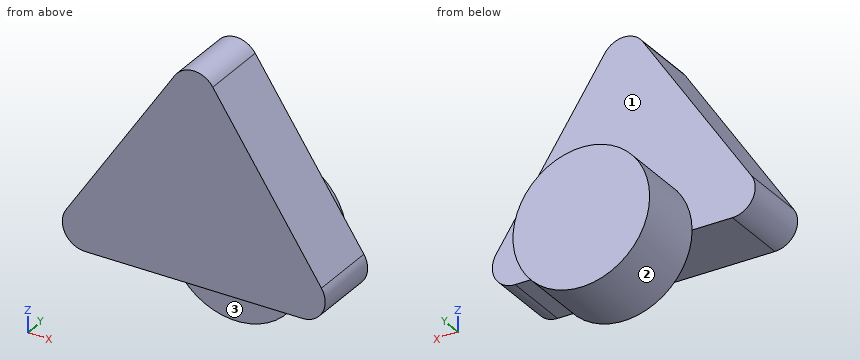
```python
from build123d import *

# Parameters (mm, degrees)
F1_DEPTH = 15
F2_R     = 15
F3_DEPTH = 15
F4_R     = 5
F5_R     = 5


with BuildPart() as f1:
    # F0 (on Front) → F1 (new body)
    with BuildSketch(Plane.XZ):
        Polygon((0, 50), (-33.166248, 0), (33.166248, 0), align=None)
    extrude(amount=F1_DEPTH)

    # F2 (on face) → F3 (join)
    with BuildSketch(Plane(origin=(0, 0, 0), x_dir=(-1, 0, 0), z_dir=(0, 1, 0))):
        Circle(F2_R)
    extrude(amount=F3_DEPTH)

    # F4
    f4_edges = [f1.edges().sort_by_distance(p)[0] for p in [
        (0, -7.5, 50),
    ]]
    fillet(f4_edges, radius=F4_R)

    # F5
    f5_edges = [f1.edges().sort_by_distance(p)[0] for p in [
        (33.166248, -7.5, 0),
        (-33.166248, -7.5, 0),
    ]]
    fillet(f5_edges, radius=F5_R)


solid = f1.part
```
CAD build for the part. Positions are in the model's coordinates, mm. Face numbers are marked on the shaded views. A direction names the side the tool comes from. Round coordinates to 2 decimals unless told otherwise and drop trailing zeros. Write each loop counter-clockwise with the first axis right and the second up, starting at its lowest first coordinate (ties: lowest second). Pieces come first, ordered by that corner, then holes. Notation, with made-up numbers: M -33.5,21.5 L 5.5,21.5 A32 cw 5.5,60.5 Z; hole C -30.5,70.25 d11. An arc over 180 degrees is marked long. One line per question, with ' | ' between items.
1. Cut at A-A on y = -12.5. Write the cut outline in (x, z).
Working result:
outline: M -28.02,7.76 A5 ccw -23.85,0 L 23.85,0 A5 ccw 28.02,7.76 L 4.17,43.72 A5 ccw -4.17,43.72 Z
2. Which spindle directions (+Z, -Z, +X, -X, +Y, -Y) get a long thin tool onto all of the face, cutting with end or side? Do the marked faces 1, 2 and 3. Say none if no direction does.
Working result:
face 1: +Z, +Y | face 2: +Y | face 3: -Z, +X, -X, -Y
3. Cut at D-D on x = -22.5. Write the cut outline in (y, z), and give its area (3 significant figures).
Working result:
outline: M -15,0 L 0,0 L 0,16.08 L -15,16.08 Z | area: 241 mm2
4. Pin check, flat tips, straight feed: pin 1 Ø4.5 at (x, y) = (7, -11) entering from -Z; pin 2 Ø10 at (y, z) = (-5.5, 27) entering from +X; pin 3 Ø10 at (y, z) = (-3.5, 3) entering from +X; pin 4 Ø3 at (x, z) = (0.5, 24.5) entering from +Y. Stop position of each tip, or through.
Working result:
pin 1: z = 0 | pin 2: x = 18.57 | pin 3: x = 28.85 | pin 4: y = 0
5. Probe L1, parallel to Y at x = -5.5, z = 38.5; L2, parallel to Y at x = 7, z = -9; L3, parallel to Z at x = 1, y = -10. List the from-to ranges inside material, lowest first. Write a range as from..to.
Working result:
L1: -15..0 | L2: 0..15 | L3: 0..45.85
6. Cut at B-B on x = 0. Write the cut outline in (y, z), and give its area (3 significant figures).
Working result:
outline: M -15,0 L 0,0 L 0,-15 L 15,-15 L 15,15 L 0,15 L 0,45.95 L -15,45.95 Z | area: 1,140 mm2
7. Cut at C-C on z = 8.5. Write the cut outline in (x, y), and give its area (3 significant figures).
Working result:
outline: M -27.53,-15 L 27.53,-15 L 27.53,0 L 12.36,0 L 12.36,15 L -12.36,15 L -12.36,0 L -27.53,0 Z | area: 1,200 mm2
